```python
from build123d import *

# Parameters (mm, degrees)
EXTRUDE1_DEPTH     = 3.175
CUT_EXTRUDE1_DEPTH = 4.175


with BuildPart() as part:
    # Sketch1 → Extrude1 (new body)
    with BuildSketch(Plane.XY):
        with BuildLine():
            Line((22.679380466, 2.841623674), (30.838674439, 7.552394246))
            ThreePointArc((30.838674439, 7.552394246), (27.49630657, 15.875), (21.959902496, 22.93087836))
            Line((21.959902496, 22.93087836), (13.800608523, 18.220107788))
            ThreePointArc((13.800608523, 18.220107788), (11.428354249, 19.794490207), (8.878771943, 21.061731462))
            Line((8.878771943, 21.061731462), (8.878771943, 30.483272606))
            ThreePointArc((8.878771943, 30.483272606), (0, 31.75), (-8.878771943, 30.483272606))
            Line((-8.878771943, 30.483272606), (-8.878771943, 21.061731462))
            ThreePointArc((-8.878771943, 21.061731462), (-11.42835425, 19.794490207), (-13.800608523, 18.220107788))
            Line((-13.800608523, 18.220107788), (-21.959902496, 22.93087836))
            ThreePointArc((-21.959902496, 22.93087836), (-27.49630657, 15.875), (-30.838674439, 7.552394246))
            Line((-30.838674439, 7.552394246), (-22.679380466, 2.841623674))
            ThreePointArc((-22.679380466, 2.841623674), (-22.856708499, 0), (-22.679380466, -2.841623674))
            Line((-22.679380466, -2.841623674), (-30.838674439, -7.552394246))
            ThreePointArc((-30.838674439, -7.552394246), (-27.49630657, -15.875), (-21.959902496, -22.93087836))
            Line((-21.959902496, -22.93087836), (-13.800608523, -18.220107788))
            ThreePointArc((-13.800608523, -18.220107788), (-11.428354249, -19.794490207), (-8.878771943, -21.061731462))
            Line((-8.878771943, -21.061731462), (-8.878771943, -30.483272606))
            ThreePointArc((-8.878771943, -30.483272606), (0, -31.75), (8.878771943, -30.483272606))
            Line((8.878771943, -30.483272606), (8.878771943, -21.061731462))
            ThreePointArc((8.878771943, -21.061731462), (11.42835425, -19.794490207), (13.800608523, -18.220107788))
            Line((13.800608523, -18.220107788), (21.959902496, -22.93087836))
            ThreePointArc((21.959902496, -22.93087836), (27.49630657, -15.875), (30.838674439, -7.552394246))
            Line((30.838674439, -7.552394246), (22.679380466, -2.841623674))
            ThreePointArc((22.679380466, -2.841623674), (22.856708499, 0), (22.679380466, 2.841623674))
        make_face()
        with BuildLine():
            Line((5.081146111, 4.229650041), (2.54665271, 2.119885858))
            ThreePointArc((2.54665271, 2.119885858), (1.656755595, 2.869584813), (0.562548705, 3.265408865))
            Line((0.562548705, 3.265408865), (1.122411451, 6.515226654))
            Line((1.122411451, 6.515226654), (3.118088913, 18.09947505))
            ThreePointArc((3.118088913, 18.09947505), (1.4e-08, 18.366095814), (-3.118088886, 18.09947505))
            Line((-3.118088886, 18.09947505), (-1.122411315, 6.515226635))
            Line((-1.122411315, 6.515226635), (-0.562548631, 3.265408874))
            ThreePointArc((-0.562548631, 3.265408874), (-1.656755527, 2.869584841), (-2.546652654, 2.119885903))
            Line((-2.546652654, 2.119885903), (-5.081146055, 4.22965016))
            Line((-5.081146055, 4.22965016), (-14.115560718, 11.750081737))
            ThreePointArc((-14.115560718, 11.750081737), (-15.90550552, 9.183047919), (-17.233649617, 6.349393341))
            Line((-17.233649617, 6.349393341), (-6.203557422, 2.285576607))
            Line((-6.203557422, 2.285576607), (-3.109201328, 1.145523033))
            ThreePointArc((-3.109201328, 1.145523033), (-3.313511107, 5e-08), (-3.109201345, -1.145522936))
            Line((-3.109201345, -1.145522936), (-6.203557501, -2.285576481))
            Line((-6.203557501, -2.285576481), (-17.233649626, -6.3493933))
            ThreePointArc((-17.233649626, -6.3493933), (-15.905505528, -9.183047878), (-14.115560727, -11.750081696))
            Line((-14.115560727, -11.750081696), (-5.081146102, -4.229650015))
            Line((-5.081146102, -4.229650015), (-2.546652687, -2.119885812))
            ThreePointArc((-2.546652687, -2.119885812), (-1.656755574, -2.869584762), (-0.562548689, -3.265408812))
            Line((-0.562548689, -3.265408812), (-1.122411442, -6.515226628))
            Line((-1.122411442, -6.515226628), (-3.118088903, -18.099475024))
            ThreePointArc((-3.118088903, -18.099475024), (-4e-09, -18.366095785), (3.118088895, -18.099475024))
            Line((3.118088895, -18.099475024), (1.122411325, -6.515226609))
            Line((1.122411325, -6.515226609), (0.562548643, -3.265408824))
            ThreePointArc((0.562548643, -3.265408824), (1.656755537, -2.869584794), (2.546652665, -2.119885861))
            Line((2.546652665, -2.119885861), (5.081146064, -4.229650134))
            Line((5.081146064, -4.229650134), (14.115560728, -11.750081711))
            ThreePointArc((14.115560728, -11.750081711), (15.905505529, -9.183047893), (17.233649627, -6.349393315))
            Line((17.233649627, -6.349393315), (6.203557431, -2.285576582))
            Line((6.203557431, -2.285576582), (3.109201343, -1.145522994))
            ThreePointArc((3.109201343, -1.145522994), (3.313511126, -1.1e-08), (3.109201368, 1.145522978))
            Line((3.109201368, 1.145522978), (6.203557511, 2.285576507))
            Line((6.203557511, 2.285576507), (17.233649636, 6.349393326))
            ThreePointArc((17.233649636, 6.349393326), (15.905505541, 9.183047906), (14.115560736, 11.750081722))
            Line((14.115560736, 11.750081722), (5.081146111, 4.229650041))
        make_face(mode=Mode.SUBTRACT)
    extrude(amount=EXTRUDE1_DEPTH)

    # Sketch2 → Cut-Extrude1 (cut, through all)
    with BuildSketch(Plane.XY.offset(3.175)):
        with BuildLine():
            Line((8.878771943, 21.061731462), (3.458150609, 8.203233505))
            ThreePointArc((3.458150609, 8.203233505), (4.451175282, 7.709661742), (5.375133304, 7.09646303))
            Line((5.375133304, 7.09646303), (13.800608523, 18.220107788))
            ThreePointArc((13.800608523, 18.220107788), (11.428354249, 19.794490207), (8.878771943, 21.061731462))
        make_face()
        with BuildLine():
            Line((22.679380466, 2.841623674), (8.833283913, 1.106770475))
            ThreePointArc((8.833283913, 1.106770475), (8.902350564, 0), (8.833283913, -1.106770475))
            Line((8.833283913, -1.106770475), (22.679380466, -2.841623674))
            ThreePointArc((22.679380466, -2.841623674), (22.856708499, 0), (22.679380466, 2.841623674))
        make_face()
        with BuildLine():
            Line((13.800608523, -18.220107788), (5.375133304, -7.09646303))
            ThreePointArc((5.375133304, -7.09646303), (4.451175282, -7.709661742), (3.458150609, -8.203233505))
            Line((3.458150609, -8.203233505), (8.878771943, -21.061731462))
            ThreePointArc((8.878771943, -21.061731462), (11.42835425, -19.794490207), (13.800608523, -18.220107788))
        make_face()
        with BuildLine():
            Line((-8.878771943, -21.061731462), (-3.458150609, -8.203233505))
            ThreePointArc((-3.458150609, -8.203233505), (-4.451175282, -7.709661742), (-5.375133304, -7.09646303))
            Line((-5.375133304, -7.09646303), (-13.800608523, -18.220107788))
            ThreePointArc((-13.800608523, -18.220107788), (-11.428354249, -19.794490207), (-8.878771943, -21.061731462))
        make_face()
        with BuildLine():
            Line((-22.679380466, -2.841623674), (-8.833283913, -1.106770475))
            ThreePointArc((-8.833283913, -1.106770475), (-8.902350564, 0), (-8.833283913, 1.106770475))
            Line((-8.833283913, 1.106770475), (-22.679380466, 2.841623674))
            ThreePointArc((-22.679380466, 2.841623674), (-22.856708499, 0), (-22.679380466, -2.841623674))
        make_face()
        with BuildLine():
            Line((-13.800608523, 18.220107788), (-5.375133304, 7.09646303))
            ThreePointArc((-5.375133304, 7.09646303), (-4.451175282, 7.709661742), (-3.458150609, 8.203233505))
            Line((-3.458150609, 8.203233505), (-8.878771943, 21.061731462))
            ThreePointArc((-8.878771943, 21.061731462), (-11.42835425, 19.794490207), (-13.800608523, 18.220107788))
        make_face()
    extrude(amount=-CUT_EXTRUDE1_DEPTH, mode=Mode.SUBTRACT)


solid = part.part
```
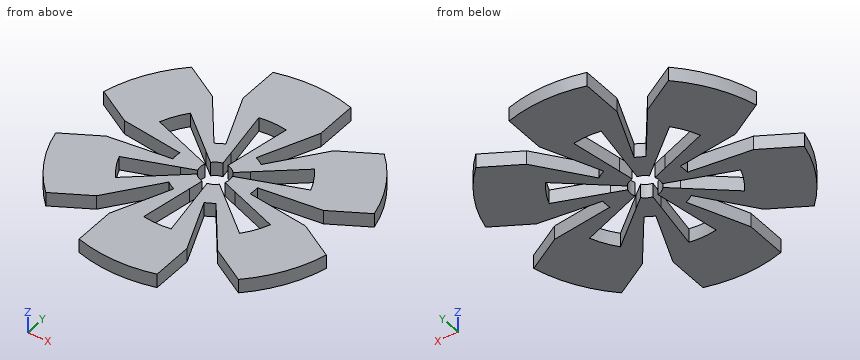
Geometry: final body of the model. Coordinates: model frame, mm. Coordinates: 2 decimals unless noted, no trailing zeros. Order: outer loops, then holes, each group sorted by start corner. A loop starts at its lowest first (then second) coordinate and runs counter-clockwise, first axis right, second up.
Item 1: Section query C-C (y = 27.5). Output: boundary loops of the cut face in (x, z) (3 decimals), then the cut area to 3 significant figures.
Answer:
outline: (-8.879, 0) - (8.879, 0) - (8.879, 3.175) - (-8.879, 3.175) - close
area: 56.4 mm2
Item 2: Material intervals for line 1 along X through (y, z) = (11, 3); line 2 along Y through (x, z) = (7, 1.85); line 3 along Y through (x, z) = (13, 2.5), sorted ascending.
Answer:
line 1: x = -29.78 to -14.71, -13.21 to -8.33, -4.64 to -1.9, 1.9 to 4.64, 8.33 to 13.21, 14.71 to 29.78
line 2: y = -30.97 to -16.61, -9.24 to -5.83, -2.58 to 2.58, 5.83 to 9.24, 16.61 to 30.97
line 3: y = -17.16 to -10.82, -4.79 to -1.63, 1.63 to 4.79, 10.82 to 17.16
Item 3: Section query A-A (x = -19.5). Output: boundary loops of the cut face in (y, z) (3 decimals), then the cut area to 3 significant figures.
Answer:
outline: (-21.511, 0) - (-2.443, 0) - (-2.443, 3.175) - (-21.511, 3.175) - close; (2.443, 0) - (21.511, 0) - (21.511, 3.175) - (2.443, 3.175) - close
area: 121 mm2
Item 4: Section query B-B (y = 11). Output: boundary loops of the cut face in (x, z) (3 decimals), then the cut area to 3 significant figures.
Answer:
outline: (-29.784, 0) - (-14.708, 0) - (-14.708, 3.175) - (-29.784, 3.175) - close; (-13.214, 0) - (-8.332, 0) - (-8.332, 3.175) - (-13.214, 3.175) - close; (-4.637, 0) - (-1.895, 0) - (-1.895, 3.175) - (-4.637, 3.175) - close; (1.895, 0) - (4.637, 0) - (4.637, 3.175) - (1.895, 3.175) - close; (8.332, 0) - (13.214, 0) - (13.214, 3.175) - (8.332, 3.175) - close; (14.708, 0) - (29.784, 0) - (29.784, 3.175) - (14.708, 3.175) - close
area: 144 mm2
Item 5: Contact query for flat-ended pins moving along their axis: P1, Ø1.5, axis at x = 24, z = 0.5, coming from the +Y side; P2, Ø1, axis at x = -24.5, z = 2.5, coming from the -Y side; P3, Ø1, axis at x = 23, z = 1, coming from the -Y side; P4, Ø12, axis at x = 12.5, y = 24, coming from the +Z side (3 decimals). Output: stop coordinate, or through.
Answer:
P1: stops at y = 21.62
P2: stops at y = -20.79
P3: stops at y = -22.4
P4: stops at z = 3.175
